Geometry check sheet. Reference: the model listing, model coordinates, mm. Face numbers are marked on the shaded views. A direction names the side the tool comes from. Round coordinates to 2 decimals unless told otherwise and drop trailing zeros. Order: outer loops, then holes, each group sorted by start corner. A loop starts at its lowest first (then second) coordinate and runs counter-clockwise, first axis right, second up. Notation, with made-up numbers: (34, 63.5) - (52, 63.5) arc R25 ccw to (52, 100.5) - close; hole circle Ø5 at (15.25, 61). An arc over 180 degrees is marked (long way). One line per question, with ' | ' between items. Start each with the question number.
Q1. Sectioned sample at A-A, the plane y = 2.1. Enter the section's corners in (x, z), then the cut area to 3 significant figures.
Q2. Tool access check on the marked faces 1, 2 and 3. Record the directions out of +Z, -Z, +X, -X, +Y, -Y that give a thin tool (end or side, any length) a straight path to the whole face; none if there is none.
Q3. Sectioned sample at B-B, the plane x = 13.5. Enter the section's corners in (y, z).
Q4. Gauge pin test, flat ends, axial feed: P1, Ø1.8, axis at x = 14.5, y = 1, coming from the +Z side; P2, Ø1, axis at x = 13, y = 3, coming from the -Z side; P3, Ø1.8, axis at x = -7.5, y = 1.5, coming from the +Z side. Record the tip position at first contact, or that the pin passes through.
Q5. Mould release check, pull along Z, two halves, no side actions. Record for the marked faces 4, 5, 6 and 7: +Z half, -Z half, draft (parallel to the pull), parting line (faces both ways), or undercut.
Q6. Material ranges on line 1 along Z through (x, y) = (-10, 2.4); line 2 along Z through (x, y) = (11, 1.7); line 3 along Z through (x, y) = (-7, 0.65), recorded low to high.
Autodesk Inventor part; units mm, degrees
ref_plane "YZ Plane" through (0, 0, 0) normal (1, 0, 0) x (0, 1, 0)
ref_plane "XZ Plane" through (0, 0, 0) normal (0, 1, 0) x (-1, 0, 0)
ref_plane "XY Plane" through (0, 0, 0) normal (0, 0, 1) x (1, 0, 0)
sketch "Sketch2" plane through (0, 0, 0) normal (0, 1, 0) x (-1, 0, 0)
  line L0 (10, -13) -> (-10, -13)
  line L1 (-13, -10) -> (-13, 10)
  line L2 (-10, 13) -> (10, 13)
  line L3 (13, 10) -> (13, -10)
  line L4 (13, -13) -> (-13, 13) construction
  line L5 (-13, -13) -> (13, 13) construction
  circle A0 centre (10, 10) radius 1.5
  circle A1 centre (-10, 10) radius 1.5
  circle A2 centre (-10, -10) radius 1.5
  circle A3 centre (10, -10) radius 1.5
  arc A4 (13, 10) -> (10, 13) centre (10, 10) ccw
  arc A5 (-10, 13) -> (-13, 10) centre (-10, 10) ccw
  arc A6 (-13, -10) -> (-10, -13) centre (-10, -10) ccw
  arc A7 (10, -13) -> (13, -10) centre (10, -10) ccw
  line L6 (13, 8.5) -> (16.5, 8.5)
  line L7 (16.5, 8.5) -> (16.5, -8.5)
  line L8 (16.5, -8.5) -> (13, -8.5)
  line L9 (13, -8.5) -> (13, 8.5)
  line L10 (0, 0) -> (6.0959, 0)
  line L11 (0, 0) -> (0, 5.3302)
  line L12 (-13, 8.5) -> (-16.5, 8.5)
  line L13 (-16.5, 8.5) -> (-16.5, -8.5)
  line L14 (-16.5, -8.5) -> (-13, -8.5)
  line L15 (-13, -8.5) -> (-13, 8.5)
  line L16 (4, 13) -> (-4, 13)
  line L17 (-4, 13) -> (-4, 16.5)
  line L18 (-4, 16.5) -> (4, 16.5)
  line L19 (4, 16.5) -> (4, 13)
  line L20 (4, -13) -> (-4, -13)
  line L21 (-4, -13) -> (-4, -16.5)
  line L22 (-4, -16.5) -> (4, -16.5)
  line L23 (4, -16.5) -> (4, -13)
  dimension "d10" = 26
  dimension "d11" = 26
  dimension "d12" = 3
  dimension "d13" = 3
  dimension "d14" = 3
  dimension "d15" = 3
  dimension "d16" = 20
  dimension "d17" = 3
  dimension "d18" = 3.5
  dimension "d19" = 17
  dimension "d20" = 8
  dimension "d21" = 3.5
extrude "Extrusion2" add sketch "Sketch2" along normal blind 3.5
properties part number "HGLRC Micro 13A 4in1 BLHeli_S"
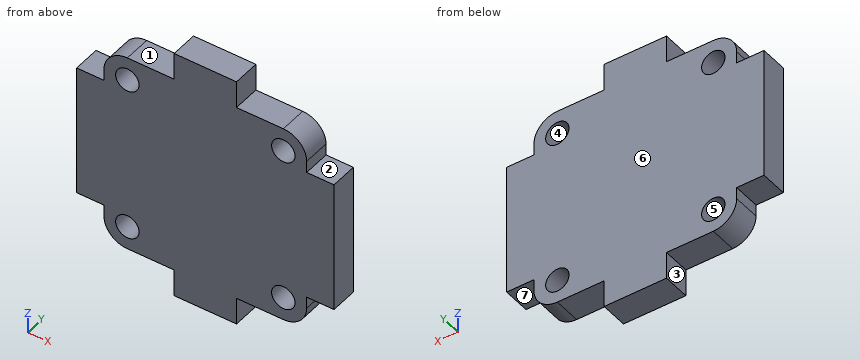
Determined:
1) outline: (-16.5, -8.5) - (-13, -8.5) - (-13, -10) arc R3 ccw to (-10, -13) - (-4, -13) - (-4, -16.5) - (4, -16.5) - (4, -13) - (10, -13) arc R3 ccw to (13, -10) - (13, -8.5) - (16.5, -8.5) - (16.5, 8.5) - (13, 8.5) - (13, 10) arc R3 ccw to (10, 13) - (4, 13) - (4, 16.5) - (-4, 16.5) - (-4, 13) - (-10, 13) arc R3 ccw to (-13, 10) - (-13, 8.5) - (-16.5, 8.5) - close; hole circle Ø3 at (-10, -10); hole circle Ø3 at (-10, 10); hole circle Ø3 at (10, -10); hole circle Ø3 at (10, 10) | area: 815 mm2
2) face 1: +Z, -X, +Y, -Y | face 2: +Z, +X, +Y, -Y | face 3: -Z, -X, +Y, -Y
3) outline: (0, -8.5) - (3.5, -8.5) - (3.5, 8.5) - (0, 8.5) - close
4) P1: stops at z = 8.5 | P2: stops at z = -11.66 | P3: stops at z = 13
5) face 4: undercut | face 5: undercut | face 6: draft | face 7: -Z half
6) line 1: z = -13 to -11.5, -8.5 to 8.5, 11.5 to 13 | line 2: z = -12.83 to -11.12, -8.88 to 8.88, 11.12 to 12.83 | line 3: z = -13 to 13
